from build123d import *

# Parameters (mm, degrees)
SKETCH1_W                   = 63.5
SKETCH1_H                   = 63.5
SKETCH1_R                   = 0.79375
SKETCH1_R_2                 = 3.5814
BOSS_EXTRUDE1_DEPTH         = 16.66875
SKETCH2_R                   = 14.732
CUT_EXTRUDE1_DEPTH          = 1.27
SKETCH3_R                   = 4.827467581
SKETCH3_R_2                 = 3.154053727
SKETCH3_R_3                 = 4.493756986
CARTIDGE_HEATER_DEPTH_DEPTH = 12.7
SKETCH4_R                   = 14.732
CUT_EXTRUDE3_DEPTH          = 12.7
CUT_EXTRUDE3_TAPER          = 47.5


with BuildPart() as part:
    # Sketch1 → Boss-Extrude1 (new body)
    with BuildSketch(Plane.XY):
        Rectangle(SKETCH1_W, SKETCH1_H)
        Circle(SKETCH1_R, mode=Mode.SUBTRACT)
        with Locations((-25.4, 25.4)):
            Circle(SKETCH1_R_2, mode=Mode.SUBTRACT)
        with Locations((25.4, 25.4)):
            Circle(SKETCH1_R_2, mode=Mode.SUBTRACT)
        with Locations((25.4, -25.4)):
            Circle(SKETCH1_R_2, mode=Mode.SUBTRACT)
        with Locations((-25.4, -25.4)):
            Circle(SKETCH1_R_2, mode=Mode.SUBTRACT)
    extrude(amount=BOSS_EXTRUDE1_DEPTH)

    # Sketch2 → Cut-Extrude1 (cut)
    with BuildSketch(Plane.XY.offset(16.66875)):
        Circle(SKETCH2_R)
    extrude(amount=-CUT_EXTRUDE1_DEPTH, mode=Mode.SUBTRACT)

    # Sketch3 → Cartidge heater (??? depth) (cut)
    with BuildSketch(Plane.ZY.offset(31.75)):
        with Locations((8.252073855, 11.1125)):
            Circle(SKETCH3_R)
        with Locations((8.252073855, 0)):
            Circle(SKETCH3_R_2)
        with Locations((8.252073855, -11.1125)):
            Circle(SKETCH3_R_3)
    extrude(amount=-CARTIDGE_HEATER_DEPTH_DEPTH, mode=Mode.SUBTRACT)

    # Sketch4 → Cut-Extrude3 (cut)
    with BuildSketch(Plane.XY.offset(15.39875)):
        Circle(SKETCH4_R)
    extrude(amount=-CUT_EXTRUDE3_DEPTH, taper=CUT_EXTRUDE3_TAPER, mode=Mode.SUBTRACT)


solid = part.part
Check sheet for the modelled part. Datum: model origin and axes. Units: mm. A direction names the side the tool comes from. Round coordinates to 2 decimals unless told otherwise and drop trailing zeros. Loops run counter-clockwise (first coordinate to the right, second up) from the corner with the lowest first, then second, coordinate; pieces in that order, holes last. Notation, with made-up numbers: M 50,-7.75 L 97,-7.75 A10 cw 97,-1.75 Z; hole C 44.25,33 d6. An arc over 180 degrees is marked long. One line per item, written item: value.
(1) Sectioned sample at B-B, the plane y = -25.4. Record the cut outline in (x, z), then the cut area to 3 significant figures.
Computed values:
outline: M -31.75,0 L -28.98,0 L -28.98,16.67 L -31.75,16.67 Z; M -21.82,0 L 21.82,0 L 21.82,16.67 L -21.82,16.67 Z; M 28.98,0 L 31.75,0 L 31.75,16.67 L 28.98,16.67 Z
area: 820 mm^2
(2) Sectioned sample at C-C, the plane z = 7.75. Record the cut outline in (x, y), then the cut area to 3 significant figures.
Computed values:
outline: M -31.75,-31.75 L 31.75,-31.75 L 31.75,31.75 L -31.75,31.75 L -31.75,15.91 L -19.05,15.91 L -19.05,6.31 L -31.75,6.31 L -31.75,3.11 L -19.05,3.11 L -19.05,-3.11 L -31.75,-3.11 L -31.75,-6.65 L -19.05,-6.65 L -19.05,-15.58 L -31.75,-15.58 Z; hole C -25.4,-25.4 d7.16; hole C -25.4,25.4 d7.16; hole C 0,0 d12.77; hole C 25.4,-25.4 d7.16; hole C 25.4,25.4 d7.16
area: 3,430 mm^2
(3) Access from +Z, -Z, +X, -X, +Y, -Y to the whole of each face (thin tool, end or side, straight path). Record for faces 4 (the face through (27.325, -22.38, 8.218)), 5 (the face through (-19.05, 0, 8)).
Computed values:
face 4: +Z, -Z
face 5: -X
(4) Sectioned sample at A-A, the plane x = -27.5. Record the cut outline in (y, z).
Computed values:
outline: M -31.75,0 L -28.3,0 L -28.3,16.67 L -31.75,16.67 Z; M -22.5,0 L 22.5,0 L 22.5,16.67 L -22.5,16.67 Z; M 28.3,0 L 31.75,0 L 31.75,16.67 L 28.3,16.67 Z; hole C -11.11,8.25 d8.99; hole C 0,8.25 d6.31; hole C 11.11,8.25 d9.65
(5) Release check for a two-part mould opening along Z. For faces 1 (the face through (-8, 15, 16.669)), 2 (the face through (-25.489, -7.323, 10.668)), 3 (the face through (27.325, 28.42, 8.218)) record: +Z half, -Z half, draft (parallel to the pull), parting line (faces both ways), or undercut.
Computed values:
face 1: +Z half
face 2: undercut
face 3: draft
(6) Thickness scan on line 1 (Y direction, x = 25.4, z = 8.75); line 2 (Y direction, x = 0, z = 2); line 3 (X direction, y = -28.5, z = 7.25). Record the ranges inside material, lowest first.
Computed values:
line 1: y = -31.75 to -28.98, -21.82 to 21.82, 28.98 to 31.75
line 2: y = -31.75 to -0.79, 0.79 to 31.75
line 3: x = -31.75 to -27.19, -23.61 to 23.61, 27.19 to 31.75
(7) Depth check by flat-ended pin: pin 1 Ø17.5 at (x, y) = (0, 0) entering from +Z; pin 2 Ø3 at (y, z) = (1, 9.5) entering from -X. Enter the tip coordinate at first touch or a pass-through.
Computed values:
pin 1: stops at z = 9.92
pin 2: stops at x = -19.05
